For this review, take the finished solid that the model builds, in its own axes (mm). Face numbers are marked on the shaded views. Coordinates: 2 decimals unless noted, no trailing zeros. Order: outer loops, then holes, each group sorted by start corner. A loop starts at its lowest first (then second) coordinate and runs counter-clockwise, first axis right, second up. Notation, with made-up numbers: (62, -0.75) -> (120, -0.75) arc R36 ccw to (120, 37.25) -> close; hole circle Ø9 at (-25, 37). An arc over 180 degrees is marked (long way). Answer as a JSON object with one key per item and string values. Group by question number.
1) Add section C-C, the plane x = 104.5. Write out the cut boundary in (y, z), then the cut area to 3 significant figures.
2) Add section A-A, the plane y = -32.5. Write out the cut boundary in (x, z).
3) For pin 1 (7 mm diameter, centred on y = 104, z = 50, fed in from +X); pin 2 (2 mm diameter, centred on x = 164, z = 22.5, fed in from +Y); pin 3 (12 mm diameter, centred on x = 244, y = 132, fed in from -Z); pin 4 (2 mm diameter, centred on x = -24.5, z = 1, fed in from +Y), all flat-tipped, find the tip position at first contact; note any pin that passes through.
4) Add section B-B, the plane y = -249.5. Write out the cut boundary in (x, z), then the cut area to 3 significant figures.
5) Draft analysis for pull direction X (two halves, no side actions). For the marked faces 1, 2, 3 and 4, state which applies: +X half, -X half, draft (parallel to the pull), parting line (faces both ways), or undercut.
6) Wall thickness on L1, parallel to Z at x = -311, y = 104; L2, parallel to X at y = 213.5, z = 73; L3, parallel to Y at x = 7.5, z = 49.5: over which ranges is each line inside the solid? List them lowest first.
from build123d import *

# Parameters (mm, degrees)
F0_W     = 624
F0_H     = 624
F1_DEPTH = 2
F2_W     = 624
F2_H     = 2
F2_W_2   = 2
F2_H_2   = 620
F3_DEPTH = 100
F4_R     = 10
F6_D     = 8
F7_W     = 422
F7_H     = 520
F8_DEPTH = 25
F9_R     = 15


with BuildPart() as f1:
    # F0 (on Top) → F1 (new body)
    with BuildSketch(Plane.XY):
        Rectangle(F0_W, F0_H)
    extrude(amount=F1_DEPTH)

    # F2 (on face) → F3 (join)
    with BuildSketch(Plane.XY.offset(2)):
        with Locations((0, -311)):
            Rectangle(F2_W, F2_H)
        with Locations((-311, 2)):
            Rectangle(F2_W_2, F2_H_2)
        with Locations((311, 2)):
            Rectangle(F2_W_2, F2_H_2)
    extrude(amount=F3_DEPTH)

    # F4
    f4_edges = [f1.edges().sort_by_distance(p)[0] for p in [
        (311, 312, 102),
        (-311, 312, 102),
        (-312, -311, 102),
        (-311, -308, 102),
        (311, -308, 102),
        (312, -311, 102),
    ]]
    fillet(f4_edges, radius=F4_R)

    # F6 (through all)
    with Locations(Plane(origin=(-312, 0, 0), x_dir=(0, -1, 0), z_dir=(-1, 0, 0))):
        with Locations((-104, 50)):
            Hole(F6_D / 2)

    # F7 (on face) → F8 (cut)
    with BuildSketch(Plane.XY.offset(2)):
        with Locations((-1, 52)):
            Rectangle(F7_W, F7_H)
    extrude(amount=-F8_DEPTH, mode=Mode.SUBTRACT)

    # F9
    f9_edges = [f1.edges().sort_by_distance(p)[0] for p in [
        (210, -208, 1),
        (210, 312, 1),
        (-212, 312, 1),
        (-212, -208, 1),
    ]]
    fillet(f9_edges, radius=F9_R)


solid = f1.part
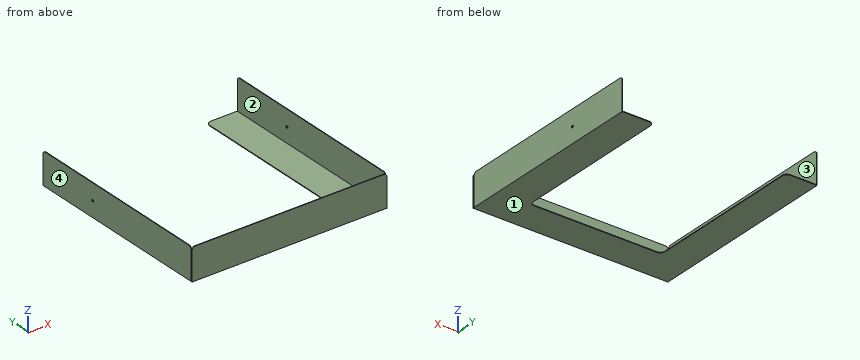
Output values:
{
 "1": {"outline": "(-312, 0) -> (-208, 0) -> (-208, 2) -> (-310, 2) -> (-310, 102) -> (-312, 102) -> close", "area": "408 mm²"},
 "2": {"outline": "(-312, 0) -> (-212, 0) -> (-212, 2) -> (-310, 2) -> (-310, 102) -> (-312, 102) -> close; (210, 0) -> (312, 0) -> (312, 102) -> (310, 102) -> (310, 2) -> (210, 2) -> close"},
 "3": {"pin 1": "passes through", "pin 2": "stops at y = -310", "pin 3": "stops at z = 0", "pin 4": "stops at y = -208"},
 "4": {"outline": "(-312, 0) -> (312, 0) -> (312, 102) -> (310, 102) -> (310, 2) -> (-310, 2) -> (-310, 102) -> (-312, 102) -> close", "area": "1,650 mm²"},
 "5": {"face 1": "draft", "face 2": "undercut", "face 3": "undercut", "face 4": "-X half"},
 "6": {"L1": "z = 0 to 46, 54 to 102", "L2": "x = -312 to -310, 310 to 312", "L3": "y = -312 to -310"}
}
